Read the model definition and answer for the solid it produces. Units are mm, in the model's axes. Face numbers are marked on the shaded views. A direction names the side the tool comes from. Give positions to 0.01 mm unless a question says otherwise; leave off trailing zeros. Loops run counter-clockwise (first coordinate to the right, second up) from the corner with the lowest first, then second, coordinate; pieces in that order, holes last.
(1) Straight lines are drawn through the part: probe 1 along Y at (x, z) = (0, -0.5); probe 2 along Z at (x, y) = (2.5, -0.5). For each, find the intervals that lie inside material, in ascending order.
(2) Find section B-B, the plane z = -0.6. Write down the section's boundary in (x, y), then the cut area to 3 significant figures.
(3) Find section A-A, the plane z = 0.1. Write down the section's boundary in (x, y).
(4) Determine the mould class of the marked faces 4, 5, 6 and 7 for opening direction X: pulls with the +X half, pulls with the -X half, needs draft (parallel to the pull), parting line crosses it, or undercut.
(5) Which of the six approach directions +Z, -Z, +X, -X, +Y, -Y give full straight-line access (tool end or side, diameter ignored) to the marked faces 1, 2 and 3?
(6) This flat-tipped pin is pushed along its axis until it touches: P1, Ø1.2, axis at x = -2.5, y = 3, coming from the +Z side. Where does it stop, or does it pass through?
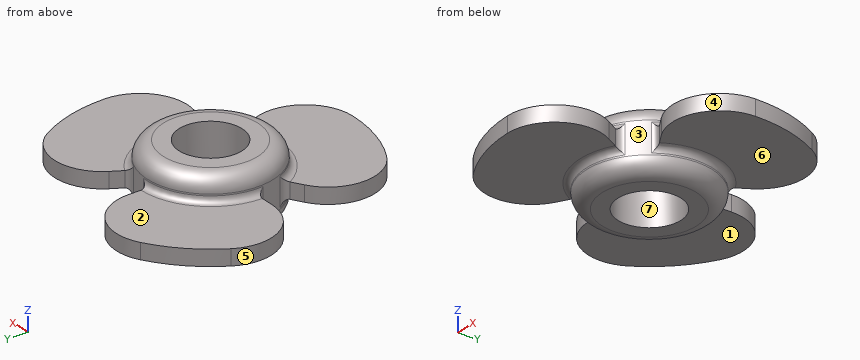
Autodesk Inventor part; units mm, degrees
ref_plane "YZ Plane" through (0, 0, 0) normal (1, 0, 0) x (0, 1, 0)
ref_plane "XZ Plane" through (0, 0, 0) normal (0, 1, 0) x (-1, 0, 0)
ref_plane "XY Plane" through (0, 0, 0) normal (0, 0, 1) x (1, 0, 0)
sketch "Sketch1" plane through (0, 0, 0) normal (0, 0, 1) x (1, 0, 0)
  circle A0 centre (0, 0) radius 2
  circle A1 centre (0, 0) radius 1
  dimension "d0" = 4
  dimension "d1" = 2
extrude "Extrusion1" add sketch "Sketch1" along normal mid plane 2
sketch "Sketch2" plane through (0, 0, 0) normal (0, 0, 1) x (1, 0, 0)
  point P0 (0, 0)
sketch "Sketch3" plane through (0, 0, 0) normal (0, 1, 0) x (-1, 0, 0)
  line L0 (2, 0.25) -> (4.5, 0.25)
  line L1 (4.5, 0.25) -> (4.5, -0.25)
  line L2 (4.5, -0.25) -> (2, -0.25)
  line L3 (2, -0.25) -> (2, 0.25)
  line L4 (2, 1) -> (-2, 1)
  line L5 (0, 0) -> (0, -2.5781)
  dimension "d4" = 0.5
  dimension "d5" = 2.5
  dimension "d6" = 0.75
  dimension "d15" = 4
revolve "Revolution1" add sketch "Sketch3" angle 90 about axis through (0, 0, 0) along (0, 0, -1)
fillet "Fillet1" radius 1.5 2 edges at (0, 4.5, 0) (-4.5, 0, 0)
fillet "Fillet2" radius 0.2 4 edges at (-2, 0, 0) (-1.4142, 1.4142, -0.25) (-1.4142, 1.4142, 0.25) (0, 2, 0)
pattern_circular "Circular Pattern1" count 3 over 360 about axis through (0, 0, 0) along (0, 0, 1) of "Revolution1", "Fillet1", "Fillet2"
fillet "Fillet3" radius 0.5 1 edges at (-2, 0, 1)
fillet "Fillet3" radius 0.5 1 edges at (-2, 0, -1)
equation "\"d1\" = 0.5 * d0"
properties part number "fan" material "PPS Plastic"
Entries:
1. probe 1: y = -2 to -1, 1 to 2
1. probe 2: z = -0.25 to 0.25
2. outline: circle Ø3.98 at (0, 0); hole circle Ø2 at (0, 0)
2. area: 9.30 mm2
3. outline: (-3.9, 2.25) arc R1.5 ccw to (-2.6, 0) - (-2.19, 0) arc R0.2 cw to (-1.99, -0.18) arc R2 ccw to (-1.82, -0.84) arc R0.2 cw to (-1.9, -1.1) - (-2.25, -1.3) arc R1.5 ccw to (-2.25, -3.9) arc R4.5 ccw to (0, -4.5) arc R1.5 ccw to (1.3, -2.25) - (1.1, -1.9) arc R0.2 cw to (1.15, -1.63) arc R2 ccw to (1.63, -1.15) arc R0.2 cw to (1.9, -1.1) - (2.25, -1.3) arc R1.5 ccw to (4.5, 0) arc R4.5 ccw to (3.9, 2.25) arc R1.5 ccw to (1.3, 2.25) - (1.1, 1.9) arc R0.2 cw to (0.84, 1.82) arc R2 ccw to (0.18, 1.99) arc R0.2 cw to (0, 2.19) - (0, 2.6) arc R1.5 ccw to (-2.25, 3.9) arc R4.5 ccw to start; hole circle Ø2 at (0, 0)
4. face 4: undercut
4. face 5: pulls with the -X half
4. face 6: needs draft
4. face 7: undercut
5. face 1: -Z, -X, +Y
5. face 2: +Z, -X, +Y
5. face 3: none
6. P1: stops at z = 0.25
